from build123d import *

# Parameters (mm, degrees)
F0_W     = 31.2911756337
F0_H     = 57.261432521
F1_DEPTH = 42.049087584
F2_W     = 35.097816959
F2_H     = 17.513435334
F3_DEPTH = 25.4
F4_T     = -2.54
F5_R     = 4.3641742047
F6_R     = 5.08


with BuildPart() as f1:
    # F0 (on Top) → F1 (new body)
    with BuildSketch(Plane.XY):
        with Locations((31.4034726471, 38.2589423098)):
            Rectangle(F0_W, F0_H)
    extrude(amount=F1_DEPTH)

    # F2 (on Right) → F3 (join)
    with BuildSketch(Plane.YZ):
        with Locations((39.5839652047, 19.7541881353)):
            Rectangle(F2_W, F2_H)
    extrude(amount=F3_DEPTH)

    # F4
    f4_openings = [f1.faces().sort_by_distance(p)[0] for p in [
        (31.403473, 38.258942, 42.049088),
    ]]
    offset(amount=F4_T, openings=f4_openings, kind=Kind.INTERSECTION)

    # F5
    f5_edges = [f1.edges().sort_by_distance(p)[0] for p in [
        (0, 39.583965, 10.99747),
    ]]
    fillet(f5_edges, radius=F5_R)

    # F6
    f6_edges = [f1.edges().sort_by_distance(p)[0] for p in [
        (0, 39.583965, 28.510906),
    ]]
    fillet(f6_edges, radius=F6_R)


solid = f1.part
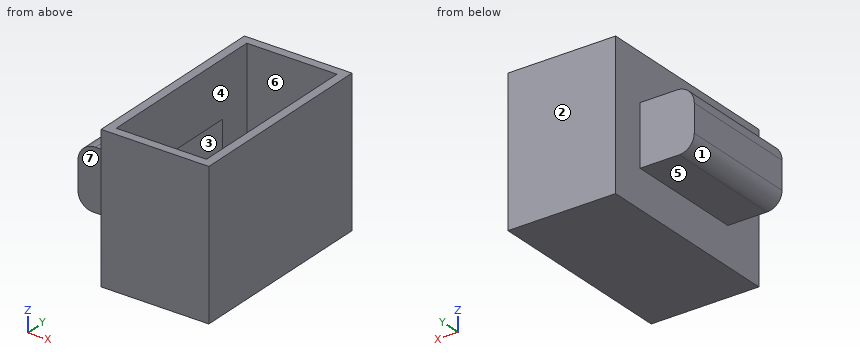
Could you check a few things on this model? Use its own coordinates, in mm. Face numbers are marked on the shaded views. A direction names the side the tool comes from. Give positions to 0.01 mm unless a question says otherwise; leave off trailing zeros. Order: outer loops, then holes, each group sorted by start corner. A loop starts at its lowest first (then second) coordinate and runs counter-clockwise, first axis right, second up.
1. Suppose I cut it at B-B (y = 20). Write out the boundary of the cut face in (x, z).
Answers below:
outline: (15.76, 0) - (47.05, 0) - (47.05, 42.05) - (44.51, 42.05) - (44.51, 2.54) - (18.3, 2.54) - (18.3, 42.05) - (15.76, 42.05) - close
2. Thinking about a two-plate mould opening in Y: for the marked faces 1, 2, 3 and 4, which applies, +Y half, -Y half, draft (parallel to the pull), parting line (faces both ways), or undercut?
Answers below:
face 1: draft
face 2: +Y half
face 3: undercut
face 4: undercut
3. I need wall thicknesses on L1, parallel to X at y = 13.5, z = 21.5; L2, parallel to Y at x = 6.5, z = 20.5; L3, parallel to Y at x = 20, z = 40. Which ranges of each line are inside material? Lowest first, please.
Answers below:
L1: x = 15.76 to 18.3, 44.51 to 47.05
L2: y = 22.04 to 24.58, 54.59 to 57.13
L3: y = 9.63 to 12.17, 64.35 to 66.89
4. Suppose I cut it at A-A (x = 13). Write out the boundary of the cut face in (y, z), plus the area to 3 significant figures.
Answers below:
outline: (22.04, 11) - (57.13, 11) - (57.13, 28.51) - (22.04, 28.51) - close; hole (24.58, 13.54) - (54.59, 13.54) - (54.59, 25.97) - (24.58, 25.97) - close
area: 241 mm2
5. Suppose I cut it at C-C (z = 37.5). Write out the boundary of the cut face in (x, y), plus the area to 3 significant figures.
Answers below:
outline: (15.76, 9.63) - (47.05, 9.63) - (47.05, 66.89) - (15.76, 66.89) - close; hole (18.3, 12.17) - (44.51, 12.17) - (44.51, 64.35) - (18.3, 64.35) - close
area: 424 mm2
6. Which directions (+Z, -Z, +X, -X, +Y, -Y) give clear straight access to the entire face, cutting with the end or side of a thin tool? Please do the marked faces 5, 6 and 7.
Answers below:
face 5: -Z, -X, +Y, -Y
face 6: +Z
face 7: +Z, -Z, -X, -Y
7. For pin 1 (3.5 mm diameter, centred on x = 11, z = 22, fed in from +Y); pin 2 (3 mm diameter, centred on x = 8.5, y = 40, fed in from -Z); pin 3 (1 mm diameter, centred on y = 15.5, z = 35.5, fed in from -X), each with a flat end and sliding along its axis, tell me the tip position at first contact or that it passes through.
Answers below:
pin 1: stops at y = 57.13
pin 2: stops at z = 11
pin 3: stops at x = 15.76
8. Suppose I cut it at D-D (x = 28). Write out the boundary of the cut face in (y, z), plus the area to 3 significant figures.
Answers below:
outline: (9.63, 0) - (66.89, 0) - (66.89, 42.05) - (64.35, 42.05) - (64.35, 2.54) - (12.17, 2.54) - (12.17, 42.05) - (9.63, 42.05) - close
area: 346 mm2
